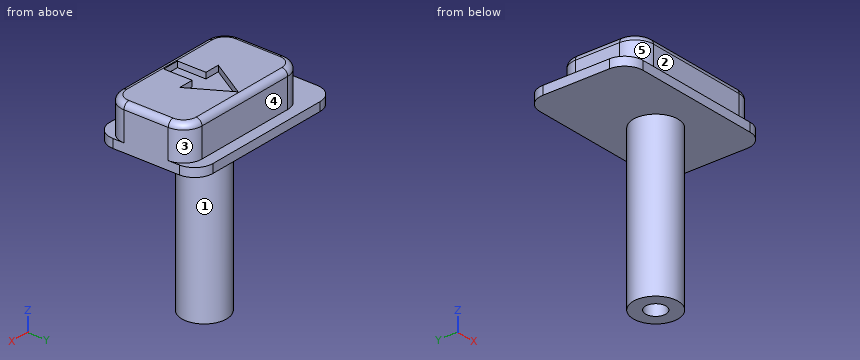
Autodesk Inventor part; units mm, degrees
ref_plane "YZ Plane" through (0, 0, 0) normal (1, 0, 0) x (0, 1, 0)
ref_plane "XZ Plane" through (0, 0, 0) normal (0, 1, 0) x (-1, 0, 0)
ref_plane "XY Plane" through (0, 0, 0) normal (0, 0, 1) x (1, 0, 0)
sketch "Sketch1" plane through (0, 0, 0) normal (0, 0, 1) x (1, 0, 0)
  circle A0 centre (0, 0) radius 1.75
  circle A1 centre (0, 0) radius 1.85
  circle A2 centre (0, 0) radius 3.85
  point P0 (0, 0)
  dimension "d0" = 0.1
  dimension "d1" = 2
extrude "Extrusion1" add sketch "Sketch1" against normal blind 5 contours A1 | A2
sketch "Sketch2" plane through (0, 0, 0) normal (0, 0, 1) x (1, 0, 0)
  point P0 (0, 0)
sketch "Sketch3" plane through (0, 0, 0) normal (0, 0, 1) x (1, 0, 0)
  circle A0 centre (0, 0) radius 3.85
extrude "Extrusion2" add sketch "Sketch3" along normal blind 22.5
sketch "Sketch4" plane through (0, 0, 22.5) normal (0, 0, 1) x (1, 0, 0)
  line L0 (12.065, -6.985) -> (-12.065, -6.985)
  line L1 (-12.065, -6.985) -> (-12.065, 6.985)
  line L2 (-12.065, 6.985) -> (12.065, 6.985)
  line L3 (12.065, 6.985) -> (12.065, -6.985)
  circle A0 centre (0, 0) radius 1.85
  line L4 (12.065, -6.985) -> (-12.065, 6.985) construction
  line L5 (-12.065, -6.985) -> (12.065, 6.985) construction
  line L6 (12.065, 12.065) -> (-12.065, 12.065) construction
  line L7 (-12.065, 12.065) -> (-12.065, 26.035) construction
  line L8 (-12.065, 26.035) -> (12.065, 26.035) construction
  line L9 (12.065, 26.035) -> (12.065, 12.065) construction
  line L10 (12.065, 12.065) -> (-12.065, 26.035) construction
  line L11 (-12.065, 12.065) -> (12.065, 26.035) construction
  line L12 (12.065, -8.89) -> (-16.51, -8.89)
  line L13 (-16.51, -8.89) -> (-16.51, 8.89)
  line L14 (-16.51, 8.89) -> (12.065, 8.89)
  line L15 (16.51, -8.89) -> (-16.51, 8.89) construction
  line L16 (-16.51, -8.89) -> (12.065, 6.4965) construction
  line L17 (12.065, -8.89) -> (12.065, 8.89)
  point P0 (0, 0)
  point P1 (0, 19.05)
  dimension "d6" = 24.13
  dimension "d7" = 13.97
  dimension "d10" = 19.05
  dimension "d16" = 17.78
extrude "Extrusion3" add sketch "Sketch4" along normal blind 1.5 contours L17 L12 L13 L14 L2 L1 L0 | L0 L1 L2 L3 | A0
extrude "Extrusion4" add sketch "Sketch4" along normal blind 7.5 contours L0 L1 L2 L3 | A0
fillet "Fillet1" radius 3.175 8 edges at (-12.065, 6.985, 27) (12.065, 6.985, 27) (12.065, -6.985, 27) (-12.065, -6.985, 27) (-16.51, -8.89, 23.25) (12.065, 8.89, 23.25) (-16.51, 8.89, 23.25) (12.065, -8.89, 23.25)
sketch "Sketch5" plane through (0, 0, 30) normal (0, 0, 1) x (1, 0, 0)
  line L0 (0, 5.8462) -> (-3.9945, -0.9035)
  line L1 (3.9945, -0.9035) -> (0, 5.8462)
  line L2 (1.4311, -0.9035) -> (1.4311, -5.8047)
  line L3 (1.4311, -5.8047) -> (-1.4311, -5.8047)
  line L4 (-1.4311, -5.8047) -> (-1.4311, -0.9035)
  line L5 (8.89, 6.985) -> (-8.89, 6.985)
  arc A0 (8.89, -6.985) -> (12.065, -3.81) centre (8.89, -3.81) ccw
  line L6 (-8.89, -6.985) -> (8.89, -6.985)
  arc A1 (-12.065, -3.81) -> (-8.89, -6.985) centre (-8.89, -3.81) ccw
  arc A2 (-8.89, 6.985) -> (-12.065, 3.81) centre (-8.89, 3.81) ccw
  line L7 (-12.065, 3.81) -> (-12.065, -3.81)
  arc A3 (12.065, 3.81) -> (8.89, 6.985) centre (8.89, 3.81) ccw
  line L8 (12.065, -3.81) -> (12.065, 3.81)
  line L9 (-3.9945, -0.9035) -> (-1.4311, -0.9035)
  line L10 (1.4311, -0.9035) -> (3.9945, -0.9035)
  point P0 (0, 0)
  point P1 (0, 0)
  point P2 (0, -0.9035)
  point P3 (0, 6.985)
emboss "Emboss1" sketch "Sketch5" operation cut depth 1 direction (0, 0, -1) contours L1 L10 L2 L3 L4 L9 L0
fillet "Fillet2" radius 1 8 edges at (-11.1351, 6.0551, 30) (-12.065, 0, 30) (-11.1351, -6.0551, 30) (0, -6.985, 30) (11.1351, -6.0551, 30) (12.065, 0, 30) (11.1351, 6.0551, 30) (0, 6.985, 30)
properties part number "Button Cover"
Verification items for the finished model (mm, model axes). Face numbers are marked on the shaded views. A direction names the side the tool comes from. Coordinates: 2 decimals unless noted, no trailing zeros. Order: outer loops, then holes, each group sorted by start corner. A loop starts at its lowest first (then second) coordinate and runs counter-clockwise, first axis right, second up. Notation, with made-up numbers: M 8.25,23.5 L 50.25,23.5 A15 ccw 50.25,28.5 Z; hole C -35,51 d10. An arc over 180 degrees is marked long. Return JSON: item names as keys, results as strings.
1) Cross-section at C-C, the plane z = 15.5. Record the boundary of the cut face in (x, y).
Answer list:
{"outline": "C 0,0 d7.7"}
2) Cross-section at B-B, the plane y = 0. Record the boundary of the cut face in (x, z) (3 decimals).
Answer list:
{"outline": "M -16.51,22.5 L -3.85,22.5 L -3.85,-5 L -1.75,-5 L -1.75,0 L 1.75,0 L 1.75,-5 L 3.85,-5 L 3.85,22.5 L 12.065,22.5 L 12.065,29 A1 ccw 11.065,30 L 3.46,30 L 3.46,29 L -3.46,29 L -3.46,30 L -11.065,30 A1 ccw -12.065,29 L -12.065,24 L -16.51,24 Z"}
3) Access from +Z, -Z, +X, -X, +Y, -Y to the whole of each face (thin tool, end or side, straight path). Record for the marked faces 1, 2, 3, 4 and 5.
Answer list:
{"face 1": "-Z", "face 2": "+Z, +X, -X, -Y", "face 3": "+Z, +X, +Y", "face 4": "+Z, +X, -X, +Y", "face 5": "+Z, -X, -Y"}
4) Cross-section at A-A, the plane x = -7.75. Record the boundary of the cut face in (y, z) (3 decimals).
Answer list:
{"outline": "M -8.89,22.5 L 8.89,22.5 L 8.89,24 L 6.985,24 L 6.985,29 A1 ccw 5.985,30 L -5.985,30 A1 ccw -6.985,29 L -6.985,24 L -8.89,24 Z"}
5) Cross-section at D-D, the plane z = -2.5. Record the boundary of the cut face in (x, y).
Answer list:
{"outline": "C 0,0 d7.7; hole C 0,0 d3.5"}
6) Gauge pin test, flat ends, axial feed: pin 1 (5.5 mm diameter, centred on x = 2.5, z = 25.5, fed in from +Y); pin 2 (10 mm diameter, centred on y = 1, z = 2.5, fed in from +X); pin 3 (10 mm diameter, centred on x = -11, z = 12, fed in from -Y); pin 4 (5 mm diameter, centred on y = -1.5, z = -1.5, fed in from -X). Record the tip position at first contact, or that the pin passes through.
Answer list:
{"pin 1": "y = 8.89", "pin 2": "x = 3.85", "pin 3": "through", "pin 4": "x = -3.85"}
7) Thickness scan on L1, parallel to Y at x = 0, z = -4; L2, parallel to Z at x = 1.25, y = 7.25; L3, parallel to Z at x = -8.25, y = 1.5. Record the ranges inside material, lowest first. Write a range as [from, to].
Answer list:
{"L1": "[-3.85, -1.75], [1.75, 3.85]", "L2": "[22.5, 24]", "L3": "[22.5, 30]"}
